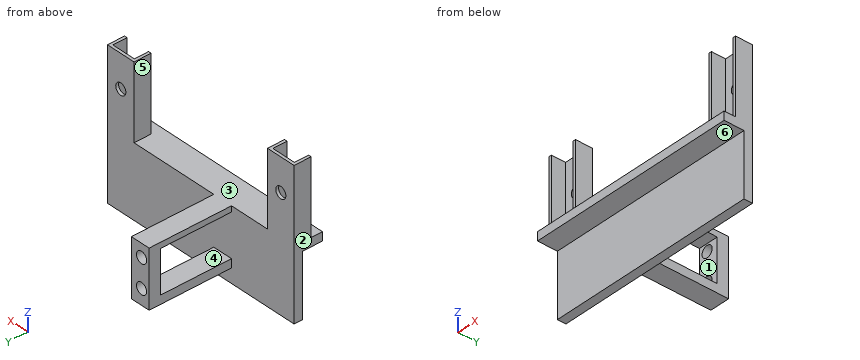
```python
from build123d import *

# Parameters (mm, degrees)
SKETCH1_W           = 73.73
SKETCH1_H           = 10
BOSS_EXTRUDE1_DEPTH = 3
BOSS_EXTRUDE2_DEPTH = 26
BOSS_EXTRUDE3_DEPTH = 26
SKETCH8_R           = 2
CUT_EXTRUDE1_DEPTH  = 80.85682751
SKETCH10_W          = 73.73
SKETCH10_H          = 3
BOSS_EXTRUDE4_DEPTH = 22
SKETCH11_W          = 7
SKETCH11_H          = 20
BOSS_EXTRUDE5_DEPTH = 29
SKETCH12_R          = 2
CUT_EXTRUDE2_DEPTH  = 10
SKETCH13_W          = 15
SKETCH13_H          = 25
CUT_EXTRUDE3_DEPTH  = 70.014491232


with BuildPart() as part:
    # Sketch1 → Boss-Extrude1 (new body)
    with BuildSketch(Plane.XY):
        with Locations((36.865, 5)):
            Rectangle(SKETCH1_W, SKETCH1_H)
    extrude(amount=BOSS_EXTRUDE1_DEPTH)

    # Sketch2 → Boss-Extrude2 (add)
    with BuildSketch(Plane.XY.offset(3)):
        Polygon((0, 4), (0, 10), (10.5, 10), (10.5, 4), (9.5, 4), (9.5, 9), (1, 9), (1, 4), align=None)
    extrude(amount=BOSS_EXTRUDE2_DEPTH)

    # Sketch7 → Boss-Extrude3 (add)
    with BuildSketch(Plane.XY.offset(3)):
        Polygon((73.73, 10), (73.73, 4), (72.73, 4), (72.73, 9), (64.23, 9), (64.23, 4), (63.23, 4), (63.23, 10), align=None)
    extrude(amount=BOSS_EXTRUDE3_DEPTH)

    # Sketch8 → Cut-Extrude1 (cut, through all)
    with BuildSketch(Plane(origin=(0, 10, 0), x_dir=(1, 0, 0), z_dir=(0, 1, 0))):
        with Locations(Location((5.25, -17.5, 0), (0, 0, 270))):
            Circle(SKETCH8_R)
        with Locations(Location((68.48, -17.5, 0), (0, 0, 270))):
            Circle(SKETCH8_R)
    extrude(amount=-CUT_EXTRUDE1_DEPTH, mode=Mode.SUBTRACT)

    # Sketch10 → Boss-Extrude4 (add)
    with BuildSketch(Plane(origin=(0, 0, 0), x_dir=(-1, 0, 0), z_dir=(0, 0, -1))):
        with Locations((-36.865, 8.5)):
            Rectangle(SKETCH10_W, SKETCH10_H)
    extrude(amount=BOSS_EXTRUDE4_DEPTH)

    # Sketch11 → Boss-Extrude5 (add)
    with BuildSketch(Plane(origin=(0, 10, 0), x_dir=(1, 0, 0), z_dir=(0, 1, 0))):
        with Locations((28.23, 7)):
            Rectangle(SKETCH11_W, SKETCH11_H)
    extrude(amount=BOSS_EXTRUDE5_DEPTH)

    # Sketch12 → Cut-Extrude2 (cut)
    with BuildSketch(Plane(origin=(0, 39, 0), x_dir=(1, 0, 0), z_dir=(0, 1, 0))):
        with Locations(Location((27.73, 11.59, 0), (0, 0, 270))):
            Circle(SKETCH12_R)
        with Locations(Location((27.73, 1.59, 0), (0, 0, 270))):
            Circle(SKETCH12_R)
    extrude(amount=-CUT_EXTRUDE2_DEPTH, mode=Mode.SUBTRACT)

    # Sketch13 → Cut-Extrude3 (cut, through all)
    with BuildSketch(Plane.ZY.offset(-24.73)):
        with Locations((-6.5, 22.5)):
            Rectangle(SKETCH13_W, SKETCH13_H)
    extrude(amount=-CUT_EXTRUDE3_DEPTH, mode=Mode.SUBTRACT)


solid = part.part
```
Model file for the job. Use its own axes, mm. Face numbers are marked on the shaded views. A direction names the side the tool comes from. Coordinates: 2 decimals unless noted, no trailing zeros. Write each loop counter-clockwise with the first axis right and the second up, starting at its lowest first coordinate (ties: lowest second). Pieces come first, ordered by that corner, then holes. Notation, with made-up numbers: (22, 21) - (68, 21) arc R9 cw to (68, 37) - close; hole circle Ø4 at (-20, 80). An arc over 180 degrees is marked (long way). One line per item, written item: value. Start each with the question number.
1. Slice it at A-A (y = 29). Write the cut outline in (x, z), plus the area to 3 significant figures.
2. Probe line 1 (X direction, y = 9.7, z = 17.5); line 2 (X direction, y = 8, z = 19); line 3 (Z direction, x = 27, y = 36). List the from-to ranges inside material, lowest first. Write a range as from..to.
3. Slice it at B-B (z = -8). Write the cut outline in (x, y).
4. Mould opens along Z. For the marked faces 1, 2 and 3 say: released by +Z, released by -Z, zero draft, split by the parting line, or undercut.
5. Slice it at C-C (x = 27.73). Write the cut outline in (y, z).
6. Flat gauge pins, fed straight in: pin 1 (7 mm diameter, centred on x = 69.5, z = 11, fed in from -Y); pin 2 (10 mm diameter, centred on y = 26.5, z = -8.5, fed in from -X); pin 3 (24 mm diameter, centred on x = 29.5, z = -10, fed in from -Y); pin 4 (5.5 mm diameter, centred on x = 29, y = 19, fed in from -Z). Where does each tip first touch, or does it go through?
7. Tool access for the marked faces 4, 5 and 6: list every direction of +Z, -Z, +X, -X, +Y, -Y with a clear straight run to the whole face (end or side of a thin tool).
8. Slice it at D-D (z = 17.5). Write the cut outline in (x, y), plus the area to 3 significant figures.
Answers below:
1. outline: (24.73, -17) - (31.73, -17) - (31.73, -14) - (24.73, -14) - close; (24.73, 1) - (31.73, 1) - (31.73, 3) - (24.73, 3) - close
1. area: 35.0 mm^2
2. line 1: x = 0..3.25, 7.25..10.5, 63.23..66.48, 70.48..73.73
2. line 2: x = 0..1, 9.5..10.5, 63.23..64.23, 72.73..73.73
2. line 3: z = -17..-13.45, -9.73..-3.45, 0.27..3
3. outline: (0, 7) - (73.73, 7) - (73.73, 10) - (0, 10) - close; (24.73, 35) - (31.73, 35) - (31.73, 39) - (24.73, 39) - close
4. face 1: undercut
4. face 2: zero draft
4. face 3: released by +Z
5. outline: (0, 0) - (7, 0) - (7, -22) - (10, -22) - (10, -17) - (39, -17) - (39, -13.59) - (35, -13.59) - (35, -14) - (10, -14) - (10, 1) - (35, 1) - (35, 0.41) - (39, 0.41) - (39, 3) - (0, 3) - close; (35, -9.59) - (39, -9.59) - (39, -3.59) - (35, -3.59) - close
6. pin 1: stops at y = 4
6. pin 2: passes through
6. pin 3: stops at y = 0
6. pin 4: stops at z = -17
7. face 4: +X, -X
7. face 5: +Z, +Y, -Y
7. face 6: -Z, +X, -X, -Y
8. outline: (0, 4) - (1, 4) - (1, 9) - (3.25, 9) - (3.25, 10) - (0, 10) - close; (7.25, 9) - (9.5, 9) - (9.5, 4) - (10.5, 4) - (10.5, 10) - (7.25, 10) - close; (63.23, 4) - (64.23, 4) - (64.23, 9) - (66.48, 9) - (66.48, 10) - (63.23, 10) - close; (70.48, 9) - (72.73, 9) - (72.73, 4) - (73.73, 4) - (73.73, 10) - (70.48, 10) - close
8. area: 33.0 mm^2
